Geometry check sheet. Reference: drawing and pictorial views, mm from the part's lowest x, y, z. A direction names the side the tool comes from. Give positions to 0.01 mm unless a question says otherwise; leave off trailing zeros. Order: outer loops, then holes, each group sorted by start corner. A loop starts at its lowest first (then second) coordinate and runs counter-clockwise, first axis right, second up. Notation, with made-up numbers: (-8.75, -36) -> (36.25, -36) arc R14 ccw to (36.25, -20) -> close; hole circle Ø7 at (72.25, 13.25). An arc over 180 degrees is marked (long way). Write each question's results on one line, items separated by ' | '.
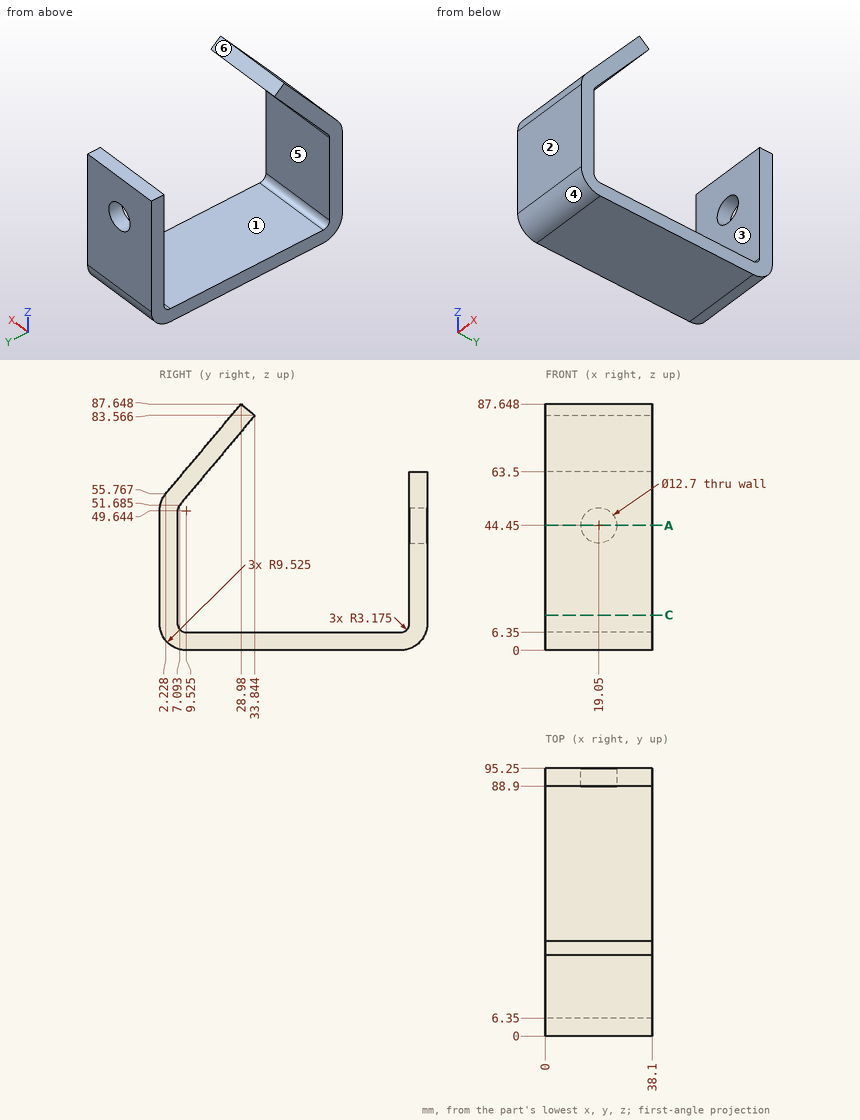
1. Section check A-A on z = 44.45. Record the cut outline in (x, y), then the cut area to 3 significant figures.
Verdict:
outline: (0, 0) -> (38.1, 0) -> (38.1, 6.35) -> (0, 6.35) -> close; (0, 88.9) -> (12.7, 88.9) -> (12.7, 95.25) -> (0, 95.25) -> close; (25.4, 88.9) -> (38.1, 88.9) -> (38.1, 95.25) -> (25.4, 95.25) -> close | area: 403 mm^2
2. Material ranges on probe 1 along Y at (x, z) = (35, 32); probe 2 along X at (y, z) = (90.75, 44.45); probe 3 along Z at (x, y) = (19.05, 94.25) (1 decimal), recorded low to high. Write a range as from..to.
Verdict:
probe 1: y = 0..6.35, 88.9..95.25 | probe 2: x = 0..12.7, 25.4..38.1 | probe 3: z = 5.3..38.1, 50.8..63.5
3. Mould release check, pull along Z, two halves, no side actions. Record for the marked faces 3, 4, 5 and 6: +Z half, -Z half, draft (parallel to the pull), parting line (faces both ways), or undercut.
Verdict:
face 3: draft | face 4: -Z half | face 5: undercut | face 6: +Z half
4. Gauge pin test, flat ends, axial feed: pin 1 Ø8 at (x, y) = (17, 10) entering from +Z (1 decimal); pin 2 Ø5 at (x, y) = (24, 91.5) entering from +Z; pin 3 Ø19 at (x, y) = (11.5, 39.5) entering from +Z. Record the tip position at first contact, or that the pin passes through.
Verdict:
pin 1: stops at z = 69.8 | pin 2: stops at z = 63.5 | pin 3: stops at z = 86.79
5. Access from +Z, -Z, +X, -X, +Y, -Y to the whole of each face (thin tool, end or side, straight path). Record for the marked faces 1 and 2.
Verdict:
face 1: +X, -X | face 2: +Z, -Z, +X, -X, -Y
6. Section check C-C on z = 12.5. Record the cut outline in (x, y), then the cut area to 3 significant figures.
Verdict:
outline: (0, 0) -> (38.1, 0) -> (38.1, 6.35) -> (0, 6.35) -> close; (0, 88.9) -> (38.1, 88.9) -> (38.1, 95.25) -> (0, 95.25) -> close | area: 484 mm^2
